```python
from build123d import *

# Parameters (mm, degrees)
SKETCH1_W           = 101.6
SKETCH1_H           = 50.8
SKETCH1_R           = 3.2639
BOSS_EXTRUDE1_DEPTH = 2.38125


with BuildPart() as part:
    # Sketch1 → Boss-Extrude1 (new, symmetric)
    with BuildSketch(Plane.XY):
        with Locations((50.8, 25.4)):
            Rectangle(SKETCH1_W, SKETCH1_H)
        with Locations(Location((12.7, 12.7, 0), (0, 0, 180))):
            Circle(SKETCH1_R, mode=Mode.SUBTRACT)
        with Locations(Location((38.1, 12.7, 0), (0, 0, 180))):
            Circle(SKETCH1_R, mode=Mode.SUBTRACT)
        with Locations(Location((63.5, 12.7, 0), (0, 0, 180))):
            Circle(SKETCH1_R, mode=Mode.SUBTRACT)
        with Locations(Location((88.9, 12.7, 0), (0, 0, 180))):
            Circle(SKETCH1_R, mode=Mode.SUBTRACT)
        with Locations(Location((12.7, 38.1, 0), (0, 0, 180))):
            Circle(SKETCH1_R, mode=Mode.SUBTRACT)
        with Locations(Location((38.1, 38.1, 0), (0, 0, 180))):
            Circle(SKETCH1_R, mode=Mode.SUBTRACT)
        with Locations(Location((63.5, 38.1, 0), (0, 0, 180))):
            Circle(SKETCH1_R, mode=Mode.SUBTRACT)
        with Locations(Location((88.9, 38.1, 0), (0, 0, 180))):
            Circle(SKETCH1_R, mode=Mode.SUBTRACT)
    extrude(amount=BOSS_EXTRUDE1_DEPTH, both=True)


solid = part.part
```
Input: part model. Units: mm. Frame: model coordinates. Give positions to 0.01 mm unless a question says otherwise; leave off trailing zeros. Order: outer loops, then holes, each group sorted by start corner. A loop starts at its lowest first (then second) coordinate and runs counter-clockwise, first axis right, second up. Notation, with made-up numbers: M -34,-4.5 L 24,-4.5 A20 ccw 24,32.5 Z; hole C 46.25,-25.5 d8. An arc over 180 degrees is marked long. Return JSON: item names as keys, results as strings.
1) Mould query, pull axis Y, two halves, no side actions, for faces 1 (the face through (50, 50.8, 0)), 2 (the face through (50, 26, 2.381)), 3 (the face through (89.608, 41.286, -0.033)), 4 (the face through (50, 0, 0)). Classes: released by +Y, released by -Y, zero draft, split by the parting line, or undercut.
Taken from the geometry:
{"face 1": "released by +Y", "face 2": "zero draft", "face 3": "undercut", "face 4": "released by -Y"}
2) Line query: L1, parallel to X at y = 38.1, z = 0; L2, parallel to X at y = 13, z = -1.9; L3, parallel to Y at x = 63.5, z = -0.2. Output: solid intervals per line, ascending. Write a range as [from, to].
Taken from the geometry:
{"L1": "x = [0, 9.44], [15.96, 34.84], [41.36, 60.24], [66.76, 85.64], [92.16, 101.6]", "L2": "x = [0, 9.45], [15.95, 34.85], [41.35, 60.25], [66.75, 85.65], [92.15, 101.6]", "L3": "y = [0, 9.44], [15.96, 34.84], [41.36, 50.8]"}
3) Section query B-B on y = 38.1. Output: boundary loops of the cut face in (x, z).
Taken from the geometry:
{"outline": "M 0,-2.38 L 9.44,-2.38 L 9.44,2.38 L 0,2.38 Z; M 15.96,-2.38 L 34.84,-2.38 L 34.84,2.38 L 15.96,2.38 Z; M 41.36,-2.38 L 60.24,-2.38 L 60.24,2.38 L 41.36,2.38 Z; M 66.76,-2.38 L 85.64,-2.38 L 85.64,2.38 L 66.76,2.38 Z; M 92.16,-2.38 L 101.6,-2.38 L 101.6,2.38 L 92.16,2.38 Z"}
4) Section query A-A on x = 12.7. Output: boundary loops of the cut face in (y, z).
Taken from the geometry:
{"outline": "M 0,-2.38 L 9.44,-2.38 L 9.44,2.38 L 0,2.38 Z; M 15.96,-2.38 L 34.84,-2.38 L 34.84,2.38 L 15.96,2.38 Z; M 41.36,-2.38 L 50.8,-2.38 L 50.8,2.38 L 41.36,2.38 Z"}
5) Section query D-D on x = 64. Output: boundary loops of the cut face in (y, z).
Taken from the geometry:
{"outline": "M 0,-2.38 L 9.47,-2.38 L 9.47,2.38 L 0,2.38 Z; M 15.93,-2.38 L 34.87,-2.38 L 34.87,2.38 L 15.93,2.38 Z; M 41.33,-2.38 L 50.8,-2.38 L 50.8,2.38 L 41.33,2.38 Z"}
6) Section query C-C on z = -0.85. Count the separate pieces of the cut face and the enclosed holes in it, and give its area (3 significant figures).
Taken from the geometry:
{"separate pieces": "1", "enclosed holes": "8", "area": "4,890 mm2"}
